Source: three-view drawing plus pictorial views. Frame: mm from the lowest corner of the part. Round coordinates to 2 decimals unless told otherwise and drop trailing zeros. Write each loop counter-clockwise with the first axis right and the second up, starting at its lowest first coordinate (ties: lowest second). Pieces come first, ordered by that corner, then holes. Notation, with made-up numbers: (8, 46) -> (63, 46) arc R11 cw to (63, 58) -> close; hole circle Ø3 at (28, 73). An arc over 180 degrees is marked (long way). Put each result on its own line as item: value.
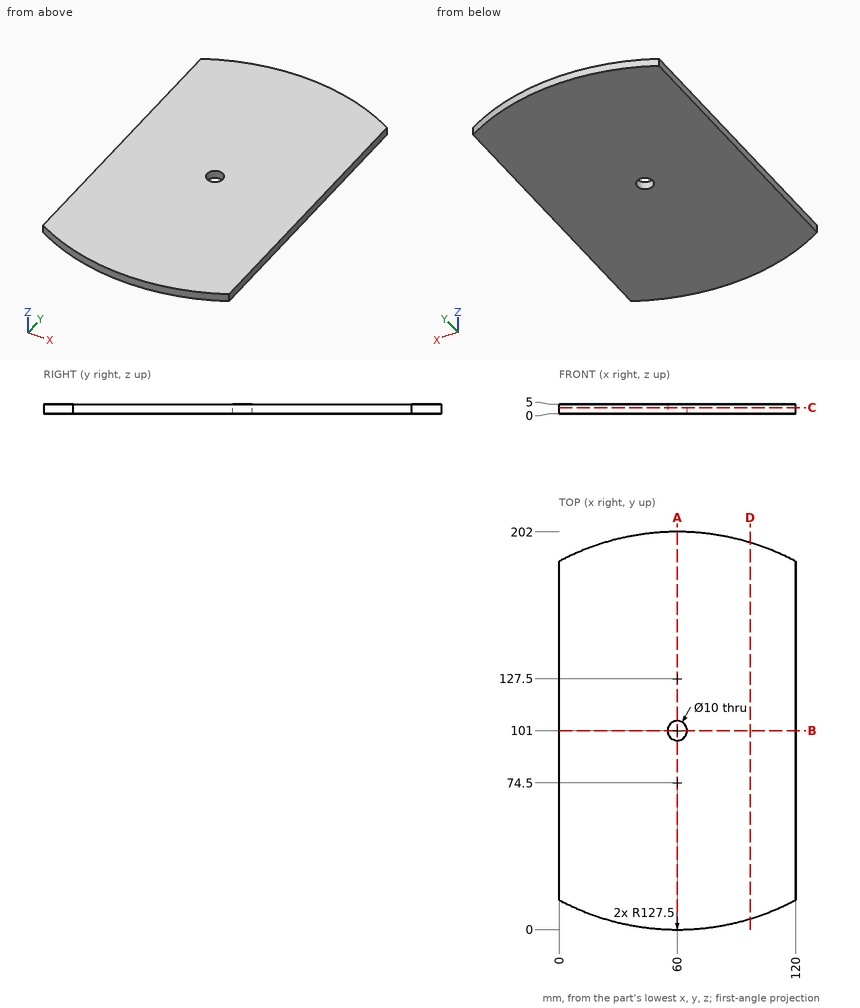
Q1. Material intervals for line 1 (Y direction, x = 60, z = 3.25); line 2 (Y direction, x = 24, z = 1.7); line 3 (Y direction, x = 50, z = 2.9), sorted ascending. Write a range as [from, to].
Ans:
line 1: y = [0, 96], [106, 202]
line 2: y = [5.19, 196.81]
line 3: y = [0.39, 201.61]
Q2. Cut plane C-C on z = 3.15. Output: boundary loops of the cut face in (x, y), and give its area (3 significant figures).
Ans:
outline: (0, 15) arc R127.5 ccw to (120, 15) -> (120, 187) arc R127.5 ccw to (0, 187) -> close; hole circle Ø10 at (60, 101)
area: 23,000 mm^2
Q3. Cut plane D-D on x = 97. Output: boundary loops of the cut face in (y, z), and give its area (3 significant figures).
Ans:
outline: (5.49, 0) -> (196.51, 0) -> (196.51, 5) -> (5.49, 5) -> close
area: 955 mm^2
Q4. Cut plane B-B on y = 101. Output: boundary loops of the cut face in (x, z), and give its area (3 significant figures).
Ans:
outline: (0, 0) -> (55, 0) -> (55, 5) -> (0, 5) -> close; (65, 0) -> (120, 0) -> (120, 5) -> (65, 5) -> close
area: 550 mm^2
Q5. Cut plane A-A on x = 60. Output: boundary loops of the cut face in (y, z).
Ans:
outline: (0, 0) -> (96, 0) -> (96, 5) -> (0, 5) -> close; (106, 0) -> (202, 0) -> (202, 5) -> (106, 5) -> close
